For this review, take the finished solid that the model builds, in its own axes (mm). A direction names the side the tool comes from. Give positions to 0.01 mm unless a question says otherwise; leave off trailing zeros. Loops run counter-clockwise (first coordinate to the right, second up) from the corner with the lowest first, then second, coordinate; pieces in that order, holes last. Notation, with made-up numbers: (60.5, 32.25) - (91.5, 32.25) arc R19 ccw to (91.5, 55.25) - close; hole circle Ø6 at (38.5, 80.25). An arc over 180 degrees is marked (long way). Answer as CSV lines item,"result".
Autodesk Inventor part; units mm, degrees
ref_plane "YZ Plane" through (0, 0, 0) normal (1, 0, 0) x (0, 1, 0)
ref_plane "XZ Plane" through (0, 0, 0) normal (0, 1, 0) x (-1, 0, 0)
ref_plane "XY Plane" through (0, 0, 0) normal (0, 0, 1) x (1, 0, 0)
sketch "Sketch1" plane through (0, 0, 0) normal (0, 0, 1) x (1, 0, 0)
  circle A0 centre (0, 0) radius 11.25
  circle A1 centre (0, 0) radius 37.0304
  arc A2 (-32.7929, -17.201) -> (-31.2929, -19.799) centre (0, 0) ccw
  line L0 (-32.7929, -17.201) -> (-31.0547, -16.1974)
  line L1 (-32.7929, -17.201) -> (-31.0547, -16.1974)
  line L2 (-29.5547, -18.7955) -> (-31.2929, -19.799)
  line L3 (-31.2929, -19.799) -> (-29.5547, -18.7955)
  line L4 (-16.1974, -31.0547) -> (-17.201, -32.7929)
  line L5 (-17.201, -32.7929) -> (-16.1974, -31.0547)
  arc A3 (-19.799, -31.2929) -> (-17.201, -32.7929) centre (0, 0) ccw
  line L6 (-19.799, -31.2929) -> (-18.7955, -29.5547)
  line L7 (-19.799, -31.2929) -> (-18.7955, -29.5547)
  arc A4 (17.201, -32.7929) -> (19.799, -31.2929) centre (0, 0) ccw
  line L8 (17.201, -32.7929) -> (16.1974, -31.0547)
  line L9 (17.201, -32.7929) -> (16.1974, -31.0547)
  line L10 (18.7955, -29.5547) -> (19.799, -31.2929)
  line L11 (19.799, -31.2929) -> (18.7955, -29.5547)
  arc A5 (31.2929, -19.799) -> (32.7929, -17.201) centre (0, 0) ccw
  line L12 (31.2929, -19.799) -> (29.5547, -18.7955)
  line L13 (31.0547, -16.1974) -> (32.7929, -17.201)
  line L14 (32.7929, -17.201) -> (31.0547, -16.1974)
  line L15 (32.7929, 17.201) -> (31.0547, 16.1974)
  line L16 (32.7929, 17.201) -> (31.0547, 16.1974)
  arc A6 (32.7929, 17.201) -> (31.2929, 19.799) centre (0, 0) ccw
  line L17 (29.5547, 18.7955) -> (31.2929, 19.799)
  line L18 (31.2929, 19.799) -> (29.5547, 18.7955)
  line L19 (16.1974, 31.0547) -> (17.201, 32.7929)
  line L20 (17.201, 32.7929) -> (16.1974, 31.0547)
  line L21 (19.799, 31.2929) -> (18.7955, 29.5547)
  line L22 (19.799, 31.2929) -> (18.7955, 29.5547)
  line L23 (-17.201, 32.7929) -> (-16.1974, 31.0547)
  line L24 (-17.201, 32.7929) -> (-16.1974, 31.0547)
  line L25 (-18.7955, 29.5547) -> (-19.799, 31.2929)
  line L26 (-19.799, 31.2929) -> (-18.7955, 29.5547)
  arc A7 (-31.2929, 19.799) -> (-32.7929, 17.201) centre (0, 0) ccw
  line L27 (-31.2929, 19.799) -> (-29.5547, 18.7955)
  line L28 (-31.2929, 19.799) -> (-29.5547, 18.7955)
  line L29 (-31.0547, 16.1974) -> (-32.7929, 17.201)
  line L30 (-32.7929, 17.201) -> (-31.0547, 16.1974)
  arc A8 (-21.806, -27.4089) -> (-27.4089, -21.806) centre (-22.4506, -22.4506) ccw
  circle A9 centre (-31.75, 0) radius 5
  arc A10 (-3.9618, 34.8002) -> (-2.3096, 31.8679) centre (-22.4506, 22.4506) ccw
  circle A11 centre (-22.4506, 22.4506) radius 5
  circle A12 centre (22.4506, 22.4506) radius 5
  circle A13 centre (22.4506, 22.4506) radius 5
  arc A14 (-3.9618, -34.8002) -> (-1.7951, -38.6456) centre (22.4506, -22.4506) ccw
  circle A15 centre (22.4506, -22.4506) radius 5
  circle A16 centre (-22.4506, 22.4506) radius 4.75
  circle A17 centre (-22.4506, -22.4506) radius 4.75
  circle A18 centre (22.4506, -22.4506) radius 4.75
  circle A19 centre (22.4506, 22.4506) radius 4.75
  circle A20 centre (0, 0) radius 34.775
  circle A21 centre (0, 0) radius 36.75
  point P0 (0, 0)
  point P1 (0, 49.75)
  point P2 (27.1463, 21.7343)
  point P3 (21.7343, 27.1463)
  point P4 (-21.7343, 27.1463)
  point P5 (-27.1463, 21.7343)
  point P6 (-27.1463, -21.7343)
  point P7 (-21.7343, -27.1463)
  point P8 (21.7343, -27.1463)
  point P9 (27.1463, -21.7343)
  dimension "d6" = 70.05
  dimension "d8" = 74.0608
  dimension "d0" = 10
  dimension "d1" = 0.25
  dimension "d4" = 360
  dimension "d7" = 0.25
  dimension "d9" = 73.5
extrude "Extrusion1" add sketch "Sketch1" along normal blind 48.3 contours A0 A10 | A9 A20 A11 A12 A15 A8 | A9 A20 A10 | A10 A20 A9 | A10 A0 | A20 A16 A11 | A8 A20 A17 | A20 A16 | A16 A20 | A20 A17 | A17 A20 | A15 A20 A18 | A20 A19 A12 | A20 A18 | A18 A20 | A20 A19 | A19 A20 picked at (-31.3962, -1.5997) picked at (-30.2693, 2.6951) picked at (-26.6756, 20.1619) picked at (20.1869, -26.6901) picked at (20.1869, 26.6901)
sketch "Skizze6" plane through (0, 0, 48.3) normal (0, 0, 1) x (1, 0, 0)
  circle A0 centre (0, 0) radius 12.225
  dimension "d33" = 24.45
extrude "Extrusion6" cut sketch "Skizze6" against normal through all
sketch "Skizze7" plane through (0, 0, 48.3) normal (0, 0, 1) x (1, 0, 0)
  line L0 (0, 0) -> (0, 1.75)
  line L1 (-25.23, 24.52) -> (25.23, 24.52)
  line L2 (25.23, 24.52) -> (25.23, -21.02)
  line L3 (25.23, -21.02) -> (-25.23, -21.02)
  line L4 (-25.23, -21.02) -> (-25.23, 24.52)
  line L5 (-25.23, 24.52) -> (25.23, -21.02) construction
  line L6 (25.23, 24.52) -> (-25.23, -21.02) construction
  dimension "d48" = 1.75
  dimension "d49" = 50.46
  dimension "d50" = 45.54
extrude "Extrusion7" cut sketch "Skizze7" against normal blind 7.4
sketch "Skizze8" plane through (0, 0, 0) normal (0, 0, -1) x (-1, 0, 0)
  circle A0 centre (0, 0) radius 12.225
  line L0 (-11.57, 11.47) -> (11.57, 11.47)
  line L1 (11.57, 11.57) -> (11.57, -11.57)
  line L2 (11.57, -11.57) -> (-11.57, -11.57)
  line L3 (-11.57, -11.57) -> (-11.57, 11.57)
  line L4 (-11.57, 11.57) -> (11.57, -11.57) construction
  line L5 (11.57, 11.57) -> (-11.57, -11.57) construction
  circle A1 centre (-11.57, 11.47) radius 1.75
  circle A2 centre (11.57, 11.47) radius 1.75
  circle A3 centre (11.57, -11.57) radius 1.75
  circle A4 centre (-11.57, -11.57) radius 1.75
  dimension "d40" = 23.14
  dimension "d41" = 23.14
  dimension "d42" = 3.5
  dimension "d43" = 3.5
  dimension "d44" = 3.5
  dimension "d45" = 3.5
extrude "Extrusion8" cut sketch "Skizze8" against normal through all contours A2 L0 L1 | L1 L0 A2 | A3 L2 L1 | L1 L2 A3 | A1 L3 L0 | L0 L3 A1 | A4 L3 L2 | L2 L3 A4
sketch "Skizze9" plane through (0, 0, 0) normal (0, 0, -1) x (-1, 0, 0)
  circle A0 centre (-11.57, 11.47) radius 1.75
  circle A1 centre (11.57, 11.47) radius 1.75
  circle A2 centre (11.57, -11.57) radius 1.75
  circle A3 centre (-11.57, -11.57) radius 1.75
  circle A4 centre (-11.57, 11.47) radius 3.1
  circle A5 centre (11.57, 11.47) radius 3.1
  circle A6 centre (11.57, -11.57) radius 3.1
  circle A7 centre (-11.57, -11.57) radius 3.1
  point P0 (0, 0)
  dimension "d51" = 6.2
  dimension "d52" = 6.2
  dimension "d53" = 6.2
  dimension "d54" = 6.2
extrude "Extrusion9" cut sketch "Skizze9" against normal blind 3.5 contours A0 | A1 | A2 | A3 | A4 | A5 | A6 | A7
properties part number "2024_09_13_beam_combiner_blende_UHP_LED"
1) Machinability: for faces 1 (the flat face through (25.23, 2, 45)), 2 (the cylindrical face through (11.95, 9.76, 21.94)), 3 (the cylindrical face through (-10.898, 8.444, 1.726)), which of the approach directions +Z, -Z, +X, -X, +Y, -Y give a long, thin tool a straight path to every point of the face, cutting with its end or side? Answer none if there is none.
From the geometry:
face 1,"+Z"
face 2,"+Z, -Z"
face 3,"-Z"
2) Consider section D-D on y = -19. Write out the cut boundary in (x, z), and give its area (3 significant figures).
From the geometry:
outline,"(-29.13, 0) - (29.13, 0) - (29.13, 48.3) - (25.23, 48.3) - (25.23, 40.9) - (-25.23, 40.9) - (-25.23, 48.3) - (-29.13, 48.3) - close"
area,"2,440 mm^2"
3) Consider section A-A on x = 0. Write out the cut boundary in (y, z) (3 decimals).
From the geometry:
outline,"(-34.775, 0) - (-12.225, 0) - (-12.225, 40.9) - (-21.02, 40.9) - (-21.02, 48.3) - (-34.775, 48.3) - close; (12.225, 0) - (34.775, 0) - (34.775, 48.3) - (24.52, 48.3) - (24.52, 40.9) - (12.225, 40.9) - close"
4) Wall thickness on line 1 (Y direction, x = -10, z = 9); line 2 (Y direction, x = -11, z = 19); line 3 (X direction, y = -11, z = 1): over which ranges is each line inside the solid? List them lowest first. Write a range as from..to.
From the geometry:
line 1,"y = -33.31..-12.34, -10.8..-7.03, 7.03..10.7, 12.24..33.31"
line 2,"y = -32.99..-13.22, -9.92..-5.33, 5.33..9.82, 13.12..32.99"
line 3,"x = -32.99..-14.62, -8.52..-5.33, 5.33..8.52, 14.62..32.99"
5) Consider section B-B on y = 0. Write out the cut boundary in (x, z) (3 decimals).
From the geometry:
outline,"(-34.775, 0) - (-12.225, 0) - (-12.225, 40.9) - (-25.23, 40.9) - (-25.23, 48.3) - (-34.775, 48.3) - close; (12.225, 0) - (34.775, 0) - (34.775, 48.3) - (25.23, 48.3) - (25.23, 40.9) - (12.225, 40.9) - close"
6) Consider section C-C on z = 38. Write out the cut boundary in (x, y) (3 decimals), and give its area (3 significant figures).
From the geometry:
outline,"(-27.146, -21.734) arc R4.75 ccw to (-21.734, -27.146) arc R34.775 ccw to (21.734, -27.146) arc R4.75 ccw to (27.146, -21.734) arc R34.775 ccw to (27.146, 21.734) arc R4.75 ccw to (21.734, 27.146) arc R34.775 ccw to (-21.734, 27.146) arc R4.75 ccw to (-27.146, 21.734) arc R34.775 ccw to start; hole circle Ø3.5 at (-11.57, -11.57); hole circle Ø3.5 at (-11.57, 11.47); hole circle Ø24.45 at (0, 0); hole circle Ø3.5 at (11.57, -11.57); hole circle Ø3.5 at (11.57, 11.47)"
area,"3,330 mm^2"
7) Insertion check: P1, Ø5, axis at x = -14.5, z = 5, coming from the -Y side; P2, Ø4.5, axis at x = 11.57, y = 11.47, coming from the +Z side; P3, Ø3, axis at x = -11.5, y = -11, coming from the -Z side. Each pin has a flat end and moves straight along its axis. Give the tip position at first contact, or say it passes through.
From the geometry:
P1,"stops at y = -32.64"
P2,"stops at z = 40.9"
P3,"stops at z = 3.5"
